The model under review builds one solid part; all positions refer to its coordinate system, in mm. A direction names the side the tool comes from. Round coordinates to 2 decimals unless told otherwise and drop trailing zeros. Write each loop counter-clockwise with the first axis right and the second up, starting at its lowest first coordinate (ties: lowest second). Pieces come first, ordered by that corner, then holes. Notation, with made-up numbers: (55.5, -38.5) - (81.5, -38.5) arc R17 cw to (81.5, -29.5) - close; hole circle Ø5 at (34, 12.25). An arc over 180 degrees is marked (long way). Return JSON: item names as keys, results as strings.
from build123d import *

# Parameters (mm, degrees)
SKETCH2_W                = 90
SKETCH2_H                = 60
BOSS_EXTRUDE1_DEPTH      = 25
SKETCH11_R               = 2.5
CUT_EXTRUDE8_DEPTH       = 5.2
SKETCH17_R               = 6.25
CUT_EXTRUDE14_DEPTH      = 2
SKETCH18_R               = 6.75
CUT_EXTRUDE15_DEPTH      = 18.8
SKETCH20_R               = 5.5
CUT_EXTRUDE17_DEPTH      = 6.21
CUT_EXTRUDE17_DEPTH_BACK = 30
SKETCH26_R               = 1.2
CUT_EXTRUDE20_DEPTH      = 62.241905284


with BuildPart() as part:
    # Sketch2 → Boss-Extrude1 (new body)
    with BuildSketch(Plane(origin=(0, 0, 0), x_dir=(1, 0, 0), z_dir=(0, 1, 0))):
        Rectangle(SKETCH2_W, SKETCH2_H)
    extrude(amount=BOSS_EXTRUDE1_DEPTH)

    # Sketch11 → Cut-Extrude8 (cut)
    with BuildSketch(Plane(origin=(0, 25, 0), x_dir=(1, 0, 0), z_dir=(0, 1, 0))):
        Circle(SKETCH11_R)
    extrude(amount=-CUT_EXTRUDE8_DEPTH, mode=Mode.SUBTRACT)

    # Sketch17 → Cut-Extrude14 (cut)
    with BuildSketch(Plane(origin=(0, 19.8, 0), x_dir=(1, 0, 0), z_dir=(0, 1, 0))):
        Circle(SKETCH17_R)
    extrude(amount=-CUT_EXTRUDE14_DEPTH, mode=Mode.SUBTRACT)

    # Sketch18 → Cut-Extrude15 (cut, through all)
    with BuildSketch(Plane(origin=(0, 17.8, 0), x_dir=(1, 0, 0), z_dir=(0, 1, 0))):
        Circle(SKETCH18_R)
    extrude(amount=-CUT_EXTRUDE15_DEPTH, mode=Mode.SUBTRACT)

    # Sketch20 → Cut-Extrude17 (cut, two sides)
    with BuildSketch(Plane(origin=(13.839745962, -7.990381057, 0), x_dir=(0, 0, 1), z_dir=(-0.866025404, 0.5, 0))) as cut_extrude17_sk:
        with Locations((0, 23)):
            Circle(SKETCH20_R)
    extrude(amount=CUT_EXTRUDE17_DEPTH, mode=Mode.SUBTRACT)
    extrude(cut_extrude17_sk.sketch, amount=-CUT_EXTRUDE17_DEPTH_BACK, mode=Mode.SUBTRACT)

    # Sketch26 → Cut-Extrude20 (cut, through all)
    with BuildSketch(Plane(origin=(8.461728205, -4.885381057, 0), x_dir=(0, 0, -1), z_dir=(0.866025404, -0.5, 0))):
        with Locations((0, 23)):
            Circle(SKETCH26_R)
    extrude(amount=-CUT_EXTRUDE20_DEPTH, mode=Mode.SUBTRACT)


solid = part.part
(1) Add section C-C (y = 13). Give the number of separate pieces and of enclosed holes in the cut face, plus the area to 3 significant figures.
Filled in:
{"separate pieces": "1", "enclosed holes": "2", "area": "5,110 mm2"}
(2) Add section A-A (x = 0). Write out the cut boundary in (y, z), plus the area to 3 significant figures.
Filled in:
{"outline": "(0, -30) - (25, -30) - (25, -2.5) - (19.8, -2.5) - (19.8, -6.25) - (17.8, -6.25) - (17.8, -6.75) - (0, -6.75) - close; (0, 6.75) - (17.8, 6.75) - (17.8, 6.25) - (19.8, 6.25) - (19.8, 2.5) - (25, 2.5) - (25, 30) - (0, 30) - close", "area": "1,210 mm2"}
(3) For faces 4 (the flat face through (45, 12, 0)), 5 (the flat face through (0, 19.8, 3)), 6 (the flat face through (19.39, 14.04, 1.15)), list the 3-axis set-ups (+Z, -Z, +X, -X, +Y, -Y) from which the entire face can be reached by the end or side of a thin tool; tool diameter is ignored.
Filled in:
{"face 4": "+Z, -Z, +X, +Y, -Y", "face 5": "-Y", "face 6": "none"}
(4) Add section B-B (z = 0). Write out the cut boundary in (x, y).
Filled in:
{"outline": "(-45, 0) - (-6.75, 0) - (-6.75, 17.8) - (-6.25, 17.8) - (-6.25, 19.8) - (-2.5, 19.8) - (-2.5, 25) - (-45, 25) - close; (2.5, 19.8) - (6.25, 19.8) - (6.25, 17.8) - (6.75, 17.8) - (6.75, 0) - (35, 0) - (17.21, 10.27) - (19.36, 13.99) - (2.5, 23.73) - close; (5.1, 25) - (20.56, 16.07) - (22.71, 19.8) - (45, 6.93) - (45, 25) - close"}
(5) Wall thickness on line 1 (Z direction, x = 0, y = 18.9); line 2 (X direction, y = 21.5, z = 0); line 3 (Z direction, x = 0, y = 21.05): over which ranges is each line inside the solid? List them lowest first.
Filled in:
{"line 1": "z = -30 to -6.25, 6.25 to 30", "line 2": "x = -45 to -2.5, 2.5 to 6.36, 11.16 to 45", "line 3": "z = -30 to -2.5, 2.5 to 30"}
(6) Mouldability with a two-part tool opening along Y and no side actions: class faces 1 (the cylindrical face through (-2.5, 22.4, -0.1)), 2 (the flat face through (-1, 0, -7)), 3 (the cylindrical face through (10.68, 19.04, 0.26)) as released by +Y, released by -Y, zero draft, split by the parting line, or undercut.
Filled in:
{"face 1": "zero draft", "face 2": "released by -Y", "face 3": "undercut"}
(7) Clearance check with a flat-ended pin moving along its axis: pin 1 Ø6 at (x, z) = (0, 0) entering from -Y. State where the tip first meets the part, or that it passes through.
Filled in:
{"pin 1": "stops at y = 19.8"}
